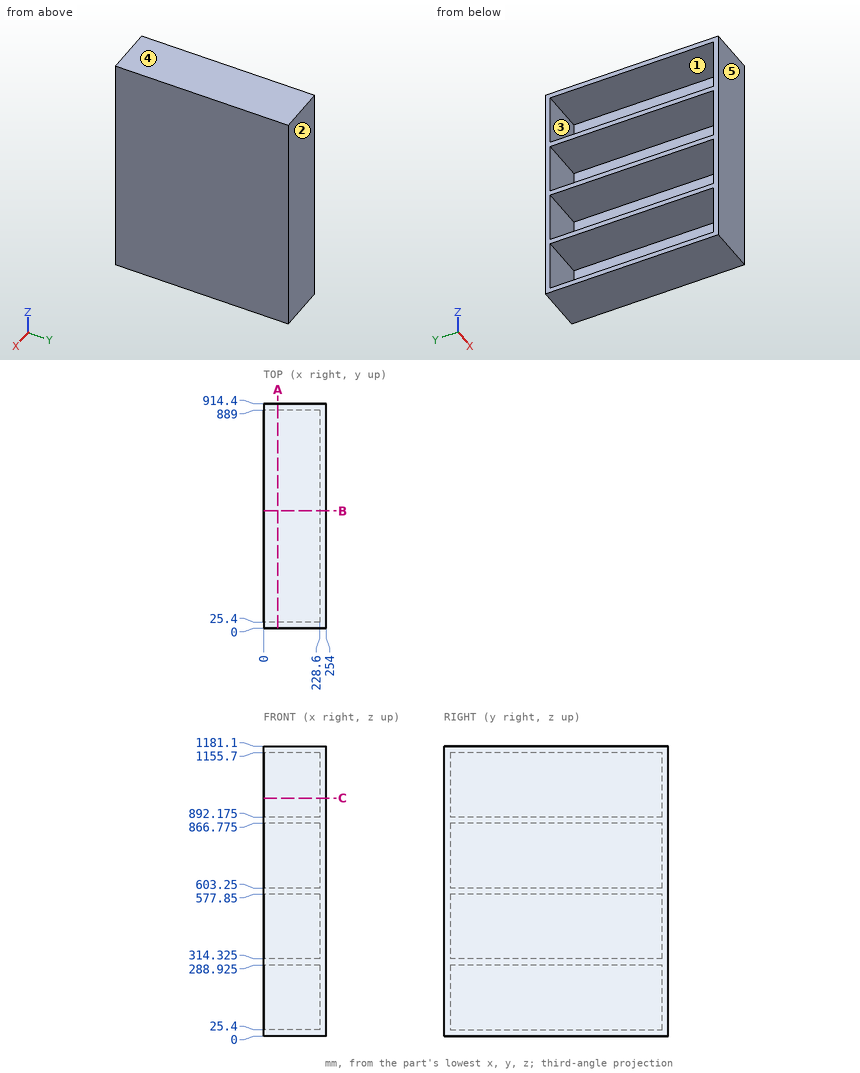
Input: dimensioned drawing with shaded views. Units: mm. Origin: part minimum x, y, z. A direction names the side the tool comes from. Round coordinates to 2 decimals unless told otherwise and drop trailing zeros. Loops run counter-clockwise (first coordinate to the right, second up) from the corner with the lowest first, then second, coordinate; pieces in that order, holes last. Notation, with made-up numbers: (27.5, 3) -> (71.5, 3) arc R11 ccw to (71.5, 13) -> close; hole circle Ø3 at (-17.5, 75.5). An arc over 180 degrees is marked (long way). Answer as a JSON object with one key per item and string values. Group by question number.
1) Section query C-C on z = 970. Output: boundary loops of the cut face in (x, y), plus the area to 3 significant figures.
2) Reachability of the marked faces 1 and 2 from +Z, -Z, +X, -X, +Y, -Y: full face, straight path, thin tool, end or side. Return the list, or none.
3) Section query A-A on x = 58. Output: boundary loops of the cut face in (y, z) (3 decimals), plus the area to 3 significant figures.
4) Ray query, L1, parallel to Z at x = 57.5, y = 304 (3 decimals); L2, parallel to Y at x = 182, z = 152.5; L3, parallel to X at y = 38.5, z = 125. Return the intervals inside material, ascending.
5) Section query B-B on y = 478.5. Output: boundary loops of the cut face in (x, z) (3 decimals).
6) Pin query (flat end, axial travel): pin 1 (3 mm diameter, centred on y = 766.5, z = 383, fed in from -X). Return the tip coordinate at first contact, or that it passes through.
7) Draft query along Z for the marked faces 3, 4 and 5. Return one class per face: +Z half, -Z half, draft (parallel to the pull), parting line (faces both ways), or undercut.
Reply:
{
 "1": {"outline": "(0, 0) -> (254, 0) -> (254, 914.4) -> (0, 914.4) -> (0, 889) -> (228.6, 889) -> (228.6, 25.4) -> (0, 25.4) -> close", "area": "34,800 mm2"},
 "2": {"face 1": "-X", "face 2": "+Z, -Z, +X, -X, +Y"},
 "3": {"outline": "(0, 0) -> (914.4, 0) -> (914.4, 1181.1) -> (0, 1181.1) -> close; hole (25.4, 25.4) -> (889, 25.4) -> (889, 288.925) -> (25.4, 288.925) -> close; hole (25.4, 314.325) -> (889, 314.325) -> (889, 577.85) -> (25.4, 577.85) -> close; hole (25.4, 603.25) -> (889, 603.25) -> (889, 866.775) -> (25.4, 866.775) -> close; hole (25.4, 892.175) -> (889, 892.175) -> (889, 1155.7) -> (25.4, 1155.7) -> close", "area": "170,000 mm2"},
 "4": {"L1": "z = 0 to 25.4, 288.925 to 314.325, 577.85 to 603.25, 866.775 to 892.175, 1155.7 to 1181.1", "L2": "y = 0 to 25.4, 889 to 914.4", "L3": "x = 228.6 to 254"},
 "5": {"outline": "(0, 0) -> (254, 0) -> (254, 1181.1) -> (0, 1181.1) -> (0, 1155.7) -> (228.6, 1155.7) -> (228.6, 892.175) -> (0, 892.175) -> (0, 866.775) -> (228.6, 866.775) -> (228.6, 603.25) -> (0, 603.25) -> (0, 577.85) -> (228.6, 577.85) -> (228.6, 314.325) -> (0, 314.325) -> (0, 288.925) -> (228.6, 288.925) -> (228.6, 25.4) -> (0, 25.4) -> close"},
 "6": {"pin 1": "stops at x = 228.6"},
 "7": {"face 3": "undercut", "face 4": "+Z half", "face 5": "draft"}
}
